```python
from build123d import *

# Parameters (mm, degrees)
BOSS_EXTRUDE1_DEPTH     = 3
CUT_EXTRUDE3_DEPTH      = 1
CUT_EXTRUDE3_DEPTH_BACK = 3
CUT_EXTRUDE4_DEPTH      = 4
SKETCH6_W               = 3
SKETCH6_H               = 30
BOSS_EXTRUDE2_DEPTH     = 20


with BuildPart() as part:
    # Sketch1 → Boss-Extrude1 (new body)
    with BuildSketch(Plane.XY):
        Polygon((-10, -15), (-10, -18), (10, -18), (10, -15), (50, -15), (50, 15), (-50, 15), (-50, -15), align=None)
    extrude(amount=BOSS_EXTRUDE1_DEPTH)

    # Sketch4 → Cut-Extrude3 (cut, two sides)
    with BuildSketch(Plane.XY.offset(3)) as cut_extrude3_sk:
        Polygon((-50, -14.220304878), (-50, -15), (1.961524227, 15), (-50, 15), align=None)
    extrude(amount=CUT_EXTRUDE3_DEPTH, mode=Mode.SUBTRACT)
    extrude(cut_extrude3_sk.sketch, amount=-CUT_EXTRUDE3_DEPTH_BACK, mode=Mode.SUBTRACT)

    # Sketch5 → Cut-Extrude4 (cut)
    with BuildSketch(Plane.XY.offset(3)):
        with BuildLine():
            Line((7.930435314, -2.338457268), (2.930435314, 6.32179677))
            ThreePointArc((2.930435314, 6.32179677), (-0.484628196, 7.236860279), (-1.399691705, 3.82179677))
            Line((-1.399691705, 3.82179677), (3.600308295, -4.838457268))
            ThreePointArc((3.600308295, -4.838457268), (7.015371804, -5.753520778), (7.930435314, -2.338457268))
        make_face()
    extrude(amount=-CUT_EXTRUDE4_DEPTH, mode=Mode.SUBTRACT)

    # Sketch6 → Boss-Extrude2 (add)
    with BuildSketch(Plane(origin=(50, 0, 0), x_dir=(0, 0, -1), z_dir=(1, 0, 0))):
        with Locations((-1.5, 0)):
            Rectangle(SKETCH6_W, SKETCH6_H)
    extrude(amount=BOSS_EXTRUDE2_DEPTH)


solid = part.part
```
Model file for the job. Use its own axes, mm. A direction names the side the tool comes from. Coordinates: 2 decimals unless noted, no trailing zeros. Write each loop counter-clockwise with the first axis right and the second up, starting at its lowest first coordinate (ties: lowest second). Pieces come first, ordered by that corner, then holes. Notation, with made-up numbers: (18.25, -3.75) - (57.25, -3.75) arc R32 cw to (57.25, 29.25) - close; hole circle Ø10 at (13, 44). An arc over 180 degrees is marked (long way). Use a Markdown table: item, result. Add a question column.
Item 1: Two-plate mould, pull along X, no slides. Class faces 4 (the face through (-10, -16, 1)), 5 (the face through (6.97, -5.78, 1.52)), 6 (the face through (70, 0, 2)), 7 (the face through (0, -18, 1)): pulls with the +X half, pulls with the -X half, needs draft (parallel to the pull), parting line crosses it, or undercut.
Item 2: Band-saw the part on C-C, the plane x = 30.5. Write the cut outline in (y, z), and give its area (3 significant figures).
Item 3: 3-axis set-ups, long thin cutter, end or side, ignore diameter. For faces 1 (the face through (1.065, -0.448, 1.521)), 2 (the face through (-30, -15, 1)), 3 (the face through (10, -17, 1)): which of +Z, -Z, +X, -X, +Y, -Y reach the whole face in a straight line?
Item 4: Band-saw the part on D-D, the plane y = 10.5. Write the cut outline in (x, z).
Item 5: Band-saw the part on A-A, the plane z = 0.5. Write the cut outline in (x, y), and give its area (3 significant figures).
Item 6: Drop a flat-ended pin along its axis: pin 1 (1 mm diameter, centred on x = 56.5, z = 2, fed in from -Y). Give the stop position or say it passes through.
Item 7: Drill centre lines: line 1 along Y through (x, z) = (4, 1.15); line 2 along Y through (x, z) = (59.5, 1.3); line 3 along X through (y, z) = (7, 2.25). Where is each one in solid material? Low to high.
Item 8: Band-saw the part on B-B, the plane y = -1. Write the cut outline in (x, z), and give its area (3 significant figures).
A:
| question | item | result |
|---|---|---|
| 1 | face 4 | pulls with the -X half |
| 1 | face 5 | undercut |
| 1 | face 6 | pulls with the +X half |
| 1 | face 7 | needs draft |
| 2 | outline | (-15, 0) - (15, 0) - (15, 3) - (-15, 3) - close |
| 2 | area | 90.0 mm² |
| 3 | face 1 | +Z, -Z |
| 3 | face 2 | +Z, -Z, -X, -Y |
| 3 | face 3 | +Z, -Z, +X, -Y |
| 4 | outline | (-5.83, 0) - (70, 0) - (70, 3) - (-5.83, 3) - close |
| 5 | outline | (-50, -15) - (-10, -15) - (-10, -18) - (10, -18) - (10, -15) - (70, -15) - (70, 15) - (1.96, 15) - close; hole (-1.4, 3.82) - (3.6, -4.84) arc R2.5 ccw to (7.93, -2.34) - (2.93, 6.32) arc R2.5 ccw to start |
| 5 | area | 2,810 mm² |
| 6 | pin 1 | stops at y = -15 |
| 7 | line 1 | y = -18 to -5.36, 4.47 to 15 |
| 7 | line 2 | y = -15 to 15 |
| 7 | line 3 | x = -11.89 to -0.83, 2.36 to 70 |
| 8 | outline | (-25.75, 0) - (1.38, 0) - (1.38, 3) - (-25.75, 3) - close; (7.16, 0) - (70, 0) - (70, 3) - (7.16, 3) - close |
| 8 | area | 270 mm² |
